Part print with two shaded views. Sizes in mm from the minimum x, y, z corner. Round coordinates to 2 decimals unless told otherwise and drop trailing zeros. Order: outer loops, then holes, each group sorted by start corner. A loop starts at its lowest first (then second) coordinate and runs counter-clockwise, first axis right, second up. Notation, with made-up numbers: M 85,55 L 133,55 A34 cw 133,94 Z; hole C 86,78 d2. An arc over 180 degrees is marked long. One line per question, with ' | ' between items.
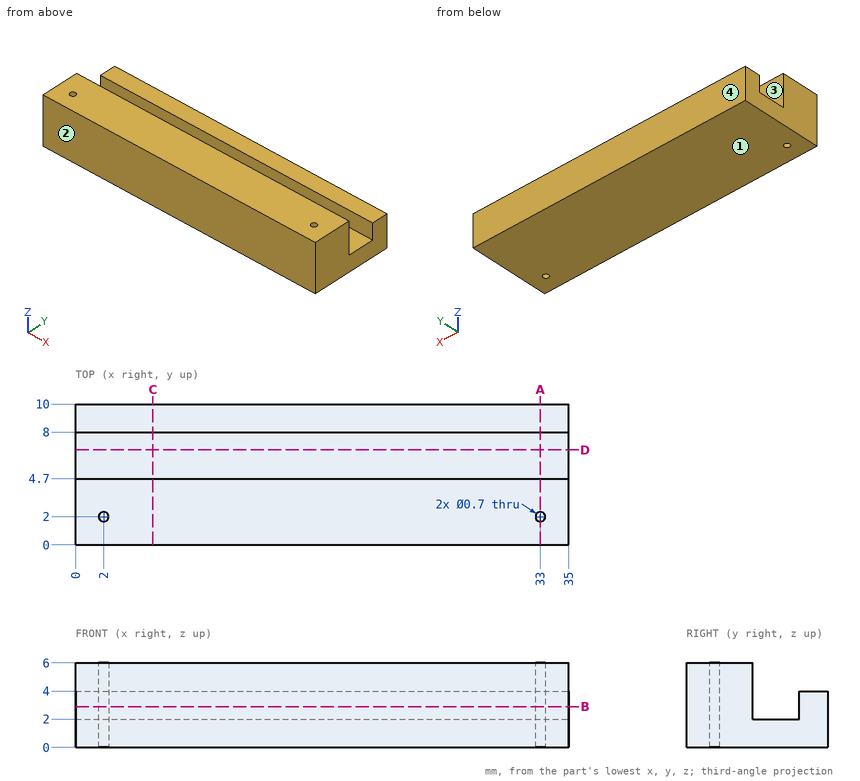
1) Two-plate mould, pull along Y, no slides. Class the marked faces 1, 2, 3 and 4: released by +Y, released by -Y, zero draft, split by the parting line, or undercut.
The answers:
face 1: zero draft | face 2: released by -Y | face 3: undercut | face 4: released by +Y
2) Saw through at D-D (y = 6.75). List the corners of the cut face in (x, z).
The answers:
outline: M 0,0 L 35,0 L 35,2 L 0,2 Z
3) Drop flat-ended pins along their axis: pin 1 (1 mm diameter, centred on x = 12, y = 9, fed in from +Z); pin 2 (1.7 mm diameter, centred on x = 14.5, y = 6, fed in from +Z). Give the stop position or say it passes through.
The answers:
pin 1: stops at z = 4 | pin 2: stops at z = 2
4) Saw through at A-A (x = 33). List the corners of the cut face in (y, z).
The answers:
outline: M 0,0 L 1.65,0 L 1.65,6 L 0,6 Z; M 2.35,0 L 10,0 L 10,4 L 8,4 L 8,2 L 4.7,2 L 4.7,6 L 2.35,6 Z
5) Saw through at C-C (x = 5.5). List the corners of the cut face in (y, z), plus the area to 3 significant figures.
The answers:
outline: M 0,0 L 10,0 L 10,4 L 8,4 L 8,2 L 4.7,2 L 4.7,6 L 0,6 Z | area: 42.8 mm²
6) Saw through at B-B (z = 2.9). List the corners of the cut face in (x, y).
The answers:
outline: M 0,0 L 35,0 L 35,4.7 L 0,4.7 Z; M 0,8 L 35,8 L 35,10 L 0,10 Z; hole C 2,2 d0.7; hole C 33,2 d0.7
7) Probe line 1 (Y direction, x = 33, z = 3.5); line 2 (Y direction, x = 2, z = 4.4); line 3 (Z direction, x = 17.5, y = 7.25). List the from-to ranges inside material, lowest first. Write a range as [from, to].
The answers:
line 1: y = [0, 1.65], [2.35, 4.7], [8, 10] | line 2: y = [0, 1.65], [2.35, 4.7] | line 3: z = [0, 2]
